CAD build for the part. Positions are in the model's coordinates, mm. A direction names the side the tool comes from. Coordinates: 2 decimals unless noted, no trailing zeros. Order: outer loops, then holes, each group sorted by start corner. A loop starts at its lowest first (then second) coordinate and runs counter-clockwise, first axis right, second up. Notation, with made-up numbers: (-33.5, 6.5) -> (19.5, 6.5) arc R12 cw to (19.5, 18.5) -> close; hole circle Ø10 at (-12.75, -11.75). An arc over 180 degrees is marked (long way). Use one line per item in the form item = value. Start each with the question number.
from build123d import *

# Parameters (mm, degrees)
SKETCH1_W           = 10
SKETCH1_H           = 10
SKETCH1_R           = 2.25
BOSS_EXTRUDE4_DEPTH = 2
BOSS_EXTRUDE5_DEPTH = 3
FILLET1_R           = 5


with BuildPart() as part:
    # Sketch1 → Boss-Extrude4 (new body)
    # profile 1 of 9: a face of its own
    with BuildSketch(Plane(origin=(0, 0, 0), x_dir=(1, 0, 0), z_dir=(0, 1, 0))):
        Polygon((70, -28), (70, 28), (58, 28), (58, 40), (-58, 40), (-58, 28), (-70, 28), (-70, -28), (-58, -28), (-58, -40), (58, -40), (58, -28), align=None)
    # profile 2 of 9: a face of its own
    with BuildSketch(Plane(origin=(0, 0, 0), x_dir=(1, 0, 0), z_dir=(0, 1, 0))):
        Polygon((-58, 28), (-58, 40), (-60, 40), (-60, 30), (-70, 30), (-70, 28), align=None)
    # profile 3 of 9: a face of its own
    with BuildSketch(Plane(origin=(0, 0, 0), x_dir=(1, 0, 0), z_dir=(0, 1, 0))):
        with Locations((-65, 35)):
            Rectangle(SKETCH1_W, SKETCH1_H)
        with Locations(Location((-65, 35, 0), (0, 0, 270))):
            Circle(SKETCH1_R, mode=Mode.SUBTRACT)
    # profile 4 of 9: a face of its own
    with BuildSketch(Plane(origin=(0, 0, 0), x_dir=(1, 0, 0), z_dir=(0, 1, 0))):
        with Locations((65, 35)):
            Rectangle(SKETCH1_W, SKETCH1_H)
        with Locations(Location((65, 35, 0), (0, 0, 270))):
            Circle(SKETCH1_R, mode=Mode.SUBTRACT)
    # profile 5 of 9: a face of its own
    with BuildSketch(Plane(origin=(0, 0, 0), x_dir=(1, 0, 0), z_dir=(0, 1, 0))):
        Polygon((70, 28), (70, 30), (60, 30), (60, 40), (58, 40), (58, 28), align=None)
    # profile 6 of 9: a face of its own
    with BuildSketch(Plane(origin=(0, 0, 0), x_dir=(1, 0, 0), z_dir=(0, 1, 0))):
        with Locations((65, -35)):
            Rectangle(SKETCH1_W, SKETCH1_H)
        with Locations(Location((65, -35, 0), (0, 0, 270))):
            Circle(SKETCH1_R, mode=Mode.SUBTRACT)
    # profile 7 of 9: a face of its own
    with BuildSketch(Plane(origin=(0, 0, 0), x_dir=(1, 0, 0), z_dir=(0, 1, 0))):
        Polygon((70, -30), (70, -28), (58, -28), (58, -40), (60, -40), (60, -30), align=None)
    # profile 8 of 9: a face of its own
    with BuildSketch(Plane(origin=(0, 0, 0), x_dir=(1, 0, 0), z_dir=(0, 1, 0))):
        Polygon((-60, -40), (-58, -40), (-58, -28), (-70, -28), (-70, -30), (-60, -30), align=None)
    # profile 9 of 9: a face of its own
    with BuildSketch(Plane(origin=(0, 0, 0), x_dir=(1, 0, 0), z_dir=(0, 1, 0))):
        with Locations((-65, -35)):
            Rectangle(SKETCH1_W, SKETCH1_H)
        with Locations(Location((-65, -35, 0), (0, 0, 270))):
            Circle(SKETCH1_R, mode=Mode.SUBTRACT)
    extrude(amount=BOSS_EXTRUDE4_DEPTH)

    # Sketch1_5 → Boss-Extrude5 (add)
    with BuildSketch(Plane(origin=(0, 0, 0), x_dir=(1, 0, 0), z_dir=(0, 1, 0))):
        Polygon((-60, -40), (-58, -40), (-58, -28), (-70, -28), (-70, -30), (-60, -30), align=None)
        Polygon((70, -30), (70, -28), (58, -28), (58, -40), (60, -40), (60, -30), align=None)
        Polygon((70, 28), (70, 30), (60, 30), (60, 40), (58, 40), (58, 28), align=None)
        Polygon((-58, 28), (-58, 40), (-60, 40), (-60, 30), (-70, 30), (-70, 28), align=None)
    extrude(amount=-BOSS_EXTRUDE5_DEPTH)

    # Fillet1
    fillet1_edges = [part.edges().sort_by_distance(p)[0] for p in [
        (70, 1, 40),
        (-70, 1, 40),
        (-70, 1, -40),
        (70, 1, -40),
    ]]
    fillet(fillet1_edges, radius=FILLET1_R)


solid = part.part
1) 3-axis set-ups, long thin cutter, end or side, ignore diameter. For faces 4 (the face through (60, -1, -35)), 5 (the face through (65, -1, 30)), 6 (the face through (-58, -1, 34)), 7 (the face through (-60, -1, -35)): which of +Z, -Z, +X, -X, +Y, -Y reach the whole face in a straight line?
2) Two-plate mould, pull along X, no slides. Class faces 1 (the face through (-67.196, 0.986, -35.488)), 2 (the face through (-1, 1, 40)), 3 (the face through (-60, -1, 35)): released by +X, released by -X, zero draft, split by the parting line, or undercut.
3) Probe L1, parallel to X at y = 0.6, z = 35; L2, parallel to Z at x = -62, y = -2.4; L3, parallel to Y at x = -47, z = 11.5. List the from-to ranges inside material, lowest first.
4) Cut at A-A on x = -8.5. Give the cut face in (y, z).
5) Cut at B-B on z = -25.5. Give the cut face in (x, y).
6) Drop flat-ended pins along their axis: P1, Ø2.5, axis at x = 66, y = -2, coming from the -Z side; P2, Ø5, axis at x = 63, z = 37, coming from the -Y side; P3, Ø3.5, axis at x = -65, z = 35, coming from the -Y side; P4, Ø2.5, axis at y = -2, z = -35.5, coming from the +X side. Give the stop position or say it passes through.
Values follow:
q1.face_4 = -Z, +X, -Y
q1.face_5 = +Z, +X, -Y
q1.face_6 = +Z, -Z, -Y
q1.face_7 = -Z, -X, -Y
q2.face_1 = undercut
q2.face_2 = zero draft
q2.face_3 = released by -X
q3.L1 = -70 to -67.25, -62.75 to 62.75, 67.25 to 70
q3.L2 = -30 to -28, 28 to 30
q3.L3 = 0 to 2
q4.outline = (0, -40) -> (2, -40) -> (2, 40) -> (0, 40) -> close
q5.outline = (-70, 0) -> (70, 0) -> (70, 2) -> (-70, 2) -> close
q6.P1 = -30
q6.P2 = 0
q6.P3 = through
q6.P4 = 60
